The listing builds one solid part. Answer for the finished solid, in the listing's coordinates (mm). Give positions to 0.01 mm unless a question says otherwise; leave off trailing zeros. Write each loop counter-clockwise with the first axis right and the second up, starting at its lowest first coordinate (ties: lowest second). Pieces come first, ordered by that corner, then holes.
```python
from build123d import *

# Parameters (mm, degrees)
SKETCH1_R             = 10
BASE_FLANGE1_DEPTH    = 2
SKETCH6_R             = 6
CUT_EXTRUDE1_DEPTH    = 15.282856857
SKETCH8_R             = 10
BASE_FLANGE2_DEPTH    = 2
SKETCH11_R            = 6
CUT_EXTRUDE2_DEPTH    = 38.416573868
SKETCH13_W            = 8
SKETCH13_H            = 3.83484861
TAB1_DEPTH            = 2
SKETCH16_W            = 8
SKETCH16_H            = 3.83484861
TAB2_DEPTH            = 2
SKETCH33_R            = 10
BOSS_EXTRUDE2_DEPTH   = 2
BOSS_EXTRUDE2_2_DEPTH = 2
BOSS_EXTRUDE2_3_DEPTH = 2
BOSS_EXTRUDE2_4_DEPTH = 2
BOSS_EXTRUDE2_5_DEPTH = 2
SKETCH23_W            = 8
SKETCH23_H            = 7.778071864
BOSS_EXTRUDE3_DEPTH   = 2
SKETCH41_R            = 6
CUT_EXTRUDE3_DEPTH    = 2


# Sheet-metal steps are written as plain solids
with BuildPart() as part:
    # Sketch1 → Base-Flange1 (new body)
    with BuildSketch(Plane(origin=(0, 0, 0), x_dir=(1, 0, 0), z_dir=(0, 1, 0))):
        with Locations(Location((0, 0, 0), (0, 0, 270))):
            Circle(SKETCH1_R)
    extrude(amount=-BASE_FLANGE1_DEPTH)

    # Sketch6 → Cut-Extrude1 (cut, through all)
    with BuildSketch(Plane(origin=(0, 0, 0), x_dir=(1, 0, 0), z_dir=(0, 1, 0))):
        with Locations(Location((0, 0, 0), (0, 0, 270))):
            Circle(SKETCH6_R)
    extrude(amount=-CUT_EXTRUDE1_DEPTH, mode=Mode.SUBTRACT)

    # Sketch13 → Tab1 (add)
    with BuildSketch(Plane(origin=(0, 0, 0), x_dir=(1, 0, 0), z_dir=(0, 1, 0))):
        with Locations((0, 11.082575695)):
            Rectangle(SKETCH13_W, SKETCH13_H)
    extrude(amount=-TAB1_DEPTH)



with BuildPart() as body_2:
    # Sketch8 → Base-Flange2 (new body)
    with BuildSketch(Plane(origin=(0, 0, 0), x_dir=(1, 0, 0), z_dir=(0, 1, 0))):
        with Locations(Location((0, 26, 0), (0, 0, 270))):
            Circle(SKETCH8_R)
    extrude(amount=-BASE_FLANGE2_DEPTH)

    # Sketch11 → Cut-Extrude2 (cut, through all)
    with BuildSketch(Plane(origin=(0, 0, 0), x_dir=(1, 0, 0), z_dir=(0, 1, 0))):
        with Locations(Location((0, 26, 0), (0, 0, 270))):
            Circle(SKETCH11_R)
    extrude(amount=-CUT_EXTRUDE2_DEPTH, mode=Mode.SUBTRACT)


with BuildPart() as part_1:
    add(part.part)

    add(body_2.part)  # Tab2 merges body 2
    # Sketch16 → Tab2 (add)
    with BuildSketch(Plane(origin=(0, 0, 0), x_dir=(1, 0, 0), z_dir=(0, 1, 0))):
        with Locations((0, 14.917424305)):
            Rectangle(SKETCH16_W, SKETCH16_H)
    extrude(amount=-TAB2_DEPTH)



with BuildPart() as body_2_2:
    # Sketch33 → Boss-Extrude2 (new body)
    with BuildSketch(Plane(origin=(0, 0, 0), x_dir=(1, 0, 0), z_dir=(0, 1, 0))):
        with Locations(Location((0, 52, 0), (0, 0, 270))):
            Circle(SKETCH33_R)
    extrude(amount=-BOSS_EXTRUDE2_DEPTH)


with BuildPart() as body_3:
    # Sketch33 → Boss-Extrude2 2 (new body)
    with BuildSketch(Plane(origin=(0, 0, 0), x_dir=(1, 0, 0), z_dir=(0, 1, 0))):
        with Locations(Location((0, 78, 0), (0, 0, 270))):
            Circle(SKETCH33_R)
    extrude(amount=-BOSS_EXTRUDE2_2_DEPTH)


with BuildPart() as body_4:
    # Sketch33 → Boss-Extrude2 3 (new body)
    with BuildSketch(Plane(origin=(0, 0, 0), x_dir=(1, 0, 0), z_dir=(0, 1, 0))):
        with Locations(Location((0, 104, 0), (0, 0, 270))):
            Circle(SKETCH33_R)
    extrude(amount=-BOSS_EXTRUDE2_3_DEPTH)


with BuildPart() as body_5:
    # Sketch33 → Boss-Extrude2 4 (new body)
    with BuildSketch(Plane(origin=(0, 0, 0), x_dir=(1, 0, 0), z_dir=(0, 1, 0))):
        with Locations(Location((0, 130, 0), (0, 0, 270))):
            Circle(SKETCH33_R)
    extrude(amount=-BOSS_EXTRUDE2_4_DEPTH)


with BuildPart() as body_6:
    # Sketch33 → Boss-Extrude2 5 (new body)
    with BuildSketch(Plane(origin=(0, 0, 0), x_dir=(1, 0, 0), z_dir=(0, 1, 0))):
        with Locations(Location((0, 179, 0), (0, 0, 270))):
            Circle(SKETCH33_R)
    extrude(amount=-BOSS_EXTRUDE2_5_DEPTH)


with BuildPart() as part_2:
    add(part_1.part)

    add(body_2_2.part)  # Boss-Extrude3 merges body 2 2

    add(body_3.part)  # Boss-Extrude3 merges body 3

    add(body_4.part)  # Boss-Extrude3 merges body 4

    add(body_5.part)  # Boss-Extrude3 merges body 5

    add(body_6.part)  # Boss-Extrude3 merges body 6
    # Sketch23 → Boss-Extrude3 (add)
    with BuildSketch(Plane(origin=(0, 0, 0), x_dir=(1, 0, 0), z_dir=(0, 1, 0))):
        with Locations((0, 39.054187322)):
            Rectangle(SKETCH23_W, SKETCH23_H)
        with Locations((0, 65.054187322)):
            Rectangle(SKETCH23_W, SKETCH23_H)
        with Locations((0, 91.054187322)):
            Rectangle(SKETCH23_W, SKETCH23_H)
        with Locations((0, 117.054187322)):
            Rectangle(SKETCH23_W, SKETCH23_H)
        Polygon((4, 139.16515139), (4, 146.943223254), (4, 160.16515139), (4, 169.043915681), (4, 173.041429596), (-4, 173.041429596), (-4, 169.043915681), (-4, 160.16515139), (-4, 146.943223254), (-4, 139.16515139), align=None)
    extrude(amount=-BOSS_EXTRUDE3_DEPTH)

    # Sketch41 → Cut-Extrude3 (cut)
    with BuildSketch(Plane(origin=(0, 0, 0), x_dir=(1, 0, 0), z_dir=(0, 1, 0))):
        with Locations(Location((0, 52, 0), (0, 0, 270))):
            Circle(SKETCH41_R)
        with Locations(Location((0, 78, 0), (0, 0, 270))):
            Circle(SKETCH41_R)
        with Locations(Location((0, 104, 0), (0, 0, 270))):
            Circle(SKETCH41_R)
        with Locations(Location((0, 130, 0), (0, 0, 270))):
            Circle(SKETCH41_R)
        with Locations(Location((0, 179, 0), (0, 0, 270))):
            Circle(SKETCH41_R)
    extrude(amount=-CUT_EXTRUDE3_DEPTH, mode=Mode.SUBTRACT)


solid = part_2.part
```
Item 1: A cutting plane is placed at D-D, the plane z = -37. Give the vertices of the cut face in (x, y).
Conclusion:
outline: (-4, -2) - (4, -2) - (4, 0) - (-4, 0) - close
Item 2: Each of these flat-tipped pins is pushed along its axis until it touches: P1, Ø1, axis at x = 0, z = -91, coming from the +Y side; P2, Ø1, axis at y = -1, z = -64.5, coming from the +X side; P3, Ø0.6, axis at y = -1, z = -115.5, coming from the -X side. Where does it stop, or does it pass through?
Conclusion:
P1: stops at y = 0
P2: stops at x = 4
P3: stops at x = -4
Item 3: A cutting plane is placed at B-B, the plane z = -130. Give the vertices of the cut face in (x, y).
Conclusion:
outline: (-10, -2) - (-6, -2) - (-6, 0) - (-10, 0) - close; (6, -2) - (10, -2) - (10, 0) - (6, 0) - close
Item 4: Determine the mould class of faces 1 (the face through (0, 0, -91)), 2 (the face through (-10, -1, -130)), 3 (the face through (10, -1, -78)) for opening direction Z: pulls with the +Z half, pulls with the -Z half, needs draft (parallel to the pull), parting line crosses it, or undercut.
Conclusion:
face 1: needs draft
face 2: undercut
face 3: undercut
Item 5: A cutting plane is placed at A-A, the plane y = -1.5. Count the separate pieces of the cut face and the enclosed holes in it, plus the area to 3 significant figures.
Conclusion:
separate pieces: 1
enclosed holes: 7
area: 1,910 mm2
Item 6: Consider probe 1 along X at (y, z) = (-1, -78); probe 2 along X at (y, z) = (-1.45, -1.5); probe 3 along X at (y, z) = (-1.5, -8). Determine where each line is inside the solid, lowest interval first.
Conclusion:
probe 1: x = -10 to -6, 6 to 10
probe 2: x = -9.89 to -5.81, 5.81 to 9.89
probe 3: x = -6 to 6
Item 7: A cutting plane is placed at C-C, the plane z = -75. Give the vertices of the cut face in (x, y), plus the area to 3 significant figures.
Conclusion:
outline: (-9.54, -2) - (-5.2, -2) - (-5.2, 0) - (-9.54, 0) - close; (5.2, -2) - (9.54, -2) - (9.54, 0) - (5.2, 0) - close
area: 17.4 mm2
